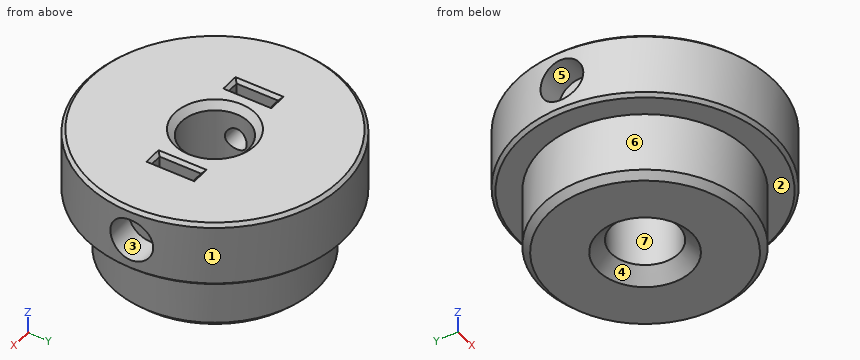
Autodesk Inventor part; units mm, degrees
ref_plane "作業平面1" through (20, 0, 0) normal (1, 0, 0) x (0, 1, 0)
ref_plane "XZ Plane" through (0, 0, 0) normal (0, 1, 0) x (-1, 0, 0)
ref_plane "XY Plane" through (0, 0, 0) normal (0, 0, 1) x (1, 0, 0)
sketch "スケッチ1" plane through (0, 0, 0) normal (0, 0, 1) x (1, 0, 0)
  circle A0 centre (0, 0) radius 15.6
  dimension "d0" = 31.2
extrude "押し出し1" add sketch "スケッチ1" along normal blind 10
sketch "スケッチ2" plane through (0, 0, 10) normal (0, 0, 1) x (1, 0, 0)
  circle A0 centre (0, 0) radius 15.6
  circle A1 centre (0, 0) radius 19.5
  dimension "d3" = 39
extrude "押し出し2" add sketch "スケッチ2" along normal blind 10 contours A0 | A1
chamfer "面取り1" distance 1 angle 45 1 edges at (-15.6, 0, 0)
chamfer "面取り2" distance 0.5 angle 45 2 edges at (-19.5, 0, 20) (-19.5, 0, 10)
sketch "スケッチ3" plane through (0, 0, 20) normal (0, 0, 1) x (1, 0, 0)
  circle A0 centre (0, 0) radius 19
  circle A1 centre (0, 0) radius 5.1
  dimension "d12" = 10.2
extrude "押し出し3" cut sketch "スケッチ3" against normal through all contours A1
chamfer "面取り3" distance 1 angle 45 1 edges at (-5.1, 0, 20)
ref_plane "作業平面1" through (20, 0, 0) normal (1, 0, 0) x (0, 1, 0)
sketch "スケッチ4" plane through (20, 0, 0) normal (1, 0, 0) x (0, 1, 0)
  line L0 (19.5, 19.5) -> (-19.5, 19.5)
  line L1 (-19.5, 10.5) -> (19.5, 10.5)
  line L2 (-19, 20) -> (19, 20)
  point P0 (0, 0)
  point P1 (0, 15)
  dimension "d44" = 5
hole "穴1" at (20, 0, 15) direction (-1, 0, 0) diameter 3.3 depth 17.75 tip angle 118
sketch "スケッチ5" plane through (20, 0, 0) normal (1, 0, 0) x (0, 1, 0)
  line L0 (-19.5, 10.5) -> (19.5, 10.5)
  line L1 (19.5, 19.5) -> (-19.5, 19.5)
  line L2 (-19, 20) -> (19, 20)
  point P0 (0, 0)
  point P1 (1.65, 15)
  point P2 (0, 15)
  point P3 (-1.65, 15)
  point P4 (1.65, 15)
  dimension "d45" = 5
hole "穴2" at (20, 0, 15) direction (-1, 0, 0) diameter 6.5 depth 5
sketch "スケッチ6" plane through (0, 0, 20) normal (0, 0, 1) x (1, 0, 0)
  circle A0 centre (0, 0) radius 19
  line L0 (8, 3.15) -> (9.8, 3.15)
  line L1 (9.8, 3.15) -> (9.8, -3.15)
  line L2 (9.8, -3.15) -> (8, -3.15)
  line L3 (8, -3.15) -> (8, 3.15)
  dimension "d34" = 1.8
  dimension "d35" = 6.3
  dimension "d36" = 3.15
  dimension "d37" = 8
extrude "押し出し4" cut sketch "スケッチ6" against normal blind 8.5 contours L0 L1 L2 L3
mirror "ミラー1" about plane through (0, 0, 0) normal (1, 0, 0) of "穴2", "穴1", "押し出し4"
chamfer "面取り4" distance 2 angle 45 1 edges at (-5.1, 0, 0)
chamfer "面取り5" distance 0.5 angle 45 8 edges at (9.8, 0, 20) (8, 0, 20) (8.9, -3.15, 20) (8.9, 3.15, 20) (-8.9, 3.15, 20) (-8.9, -3.15, 20) (-9.8, 0, 20) (-8, 0, 20)
properties part number "Print_Parts_A1" material "PC/ABS プラスチック"
The listing builds one solid part. Answer for the finished solid, in the listing's coordinates (mm). Face numbers are marked on the shaded views. A direction names the side the tool comes from. Give positions to 0.01 mm unless a question says otherwise; leave off trailing zeros. Write each loop counter-clockwise with the first axis right and the second up, starting at its lowest first coordinate (ties: lowest second). Pieces come first, ordered by that corner, then holes.
1) For a pull along X with two mould halves and no side action, classify the marked faces 4, 5, 6 and 7 as pulls with the +X half, pulls with the -X half, needs draft (parallel to the pull), parting line crosses it, or undercut.
2) Section D-D (z = 8) is taken. Write down the section's boundary in (x, y).
3) Section C-C (y = 0) is taken. Count the separate pieces of the cut face and the enclosed holes in it, and give its area (3 significant figures).
4) Section A-A (x = 0) is taken. Write down the section's boundary in (y, z).
5) A tool of negligible diameter and unlimited length cuts with its end or side. For the marked faces 1, 2 and 3, from which of +Z, -Z, +X, -X, +Y, -Y can it reach the whole face along a straight path? Write none if from no direction.
6) Given P1, Ø3, axis at y = 0, z = 15, coming from the +X side; P2, Ø1, axis at x = 1.5, z = 17.5, coming from the -Y side; P3, Ø5.5, axis at y = 0, z = 15, coming from the -X side; P4, Ø2, axis at x = 9, z = 16, coming from the +Y side, each flat-ended and moving along its own axis, determine where each tip first touches the part or whether it passes through.
7) Find the intervals of material crossed by L1, parallel to Z at x = 11.85, y = 0; L2, parallel to Z at x = 14, y = 9; L3, parallel to X at y = 2, z = 16.75, in increasing order.
Response:
1. face 4: undercut
1. face 5: needs draft
1. face 6: parting line crosses it
1. face 7: undercut
2. outline: circle Ø31.2 at (0, 0); hole circle Ø10.2 at (0, 0)
3. separate pieces: 6
3. enclosed holes: 0
3. area: 348 mm2
4. outline: (-19.5, 10.5) - (-19, 10) - (-15.6, 10) - (-15.6, 1) - (-14.6, 0) - (-7.1, 0) - (-5.1, 2) - (-5.1, 19) - (-6.1, 20) - (-19, 20) - (-19.5, 19.5) - close; (5.1, 2) - (7.1, 0) - (14.6, 0) - (15.6, 1) - (15.6, 10) - (19, 10) - (19.5, 10.5) - (19.5, 19.5) - (19, 20) - (6.1, 20) - (5.1, 19) - close
5. face 1: +Z, -Z
5. face 2: -Z
5. face 3: +X
6. P1: passes through
6. P2: stops at y = -19.47
6. P3: stops at x = -15
6. P4: stops at y = 17.78
7. L1: z = 0 to 13.35, 16.65 to 20
7. L2: z = 10 to 20
7. L3: x = -15 to -9.8, -8 to -4.69, 4.69 to 8, 9.8 to 15
